The listing builds one solid part. Answer for the finished solid, in the listing's coordinates (mm). A direction names the side the tool comes from. Coordinates: 2 decimals unless noted, no trailing zeros. Loops run counter-clockwise (first coordinate to the right, second up) from the corner with the lowest first, then second, coordinate; pieces in that order, holes last. Notation, with made-up numbers: (-39.75, 73) - (-21.75, 73) arc R31 ccw to (-21.75, 109) - close; hole circle Ø10 at (-22.5, -10). An arc over 180 degrees is marked (long way). One line per question, with ' | ' between items.
from build123d import *

# Parameters (mm, degrees)
SKETCH_1_R      = 5
EXTRUDE_1_DEPTH = 10
CHAMFER_1_SIZE  = 1
SKETCH_2_R      = 4
EXTRUDE_2_DEPTH = 30
SKETCH_3_R      = 2
EXTRUDE_3_DEPTH = 10
FILLET_1_R      = 2


with BuildPart() as part:
    # Эскиз1 → Бобышка-Вытянуть1 (new body)
    with BuildSketch(Plane.XY):
        Circle(SKETCH_1_R)
    extrude(amount=EXTRUDE_1_DEPTH)

    # Фаска1
    chamfer_1_edges = [part.edges().sort_by_distance(p)[0] for p in [
        (-5, 0, 10),
    ]]
    chamfer(chamfer_1_edges, length=CHAMFER_1_SIZE)

    # Эскиз2 → Бобышка-Вытянуть2 (add)
    with BuildSketch(Plane.XY.offset(10)):
        Circle(SKETCH_2_R)
    extrude(amount=EXTRUDE_2_DEPTH)

    # Эскиз3 → Бобышка-Вытянуть3 (add)
    with BuildSketch(Plane.XY.offset(40)):
        Circle(SKETCH_3_R)
    extrude(amount=EXTRUDE_3_DEPTH)

    # Скругление1
    fillet_1_edges = [part.edges().sort_by_distance(p)[0] for p in [
        (-2, 0, 50),
    ]]
    fillet(fillet_1_edges, radius=FILLET_1_R)


solid = part.part
Item 1: Which of the six approach directions +Z, -Z, +X, -X, +Y, -Y give full straight-line access (tool end or side, diameter ignored) to faces 1 (the face through (0, -2, 44)), 2 (the face through (-1.08, -4.88, 4.44))?
Taken from the geometry:
face 1: +Z | face 2: +Z, -Z
Item 2: Find section A-A, the plane x = 0. Write down the section's boundary in (y, z), plus the area to 3 significant figures.
Taken from the geometry:
outline: (-5, 0) - (5, 0) - (5, 9) - (4, 10) - (4, 40) - (2, 40) - (2, 48) arc R2 ccw to (-2, 48) - (-2, 40) - (-4, 40) - (-4, 10) - (-5, 9) - close | area: 377 mm2
Item 3: Find the intervals of material crossed by line 1 (Z direction, x = 2, y = -3.25); line 2 (Y direction, x = 0, z = 16); line 3 (Y direction, x = 2.75, z = 4), in increasing order. Write a range as [from, to].
Taken from the geometry:
line 1: z = [0, 40] | line 2: y = [-4, 4] | line 3: y = [-4.18, 4.18]
Item 4: Each of these flat-tipped pins is pushed along its axis until it touches: pin 1 Ø3 at (x, z) = (-3.5, 31.5) entering from +Y; pin 2 Ø5 at (y, z) = (2, 11.5) entering from +X; pin 3 Ø1.5 at (y, z) = (-1, 13) entering from -X. Where does it stop, or does it pass through?
Taken from the geometry:
pin 1: stops at y = 3.46 | pin 2: stops at x = 4.72 | pin 3: stops at x = -3.99
Item 5: Find section B-B, the plane z = 11.5. Write down the section's boundary in (x, y), plus the area to 3 significant figures.
Taken from the geometry:
outline: circle Ø8 at (0, 0) | area: 50.3 mm2
Item 6: Find section C-C, the plane z = 5.5. Write down the section's boundary in (x, y), plus the area to 3 significant figures.
Taken from the geometry:
outline: circle Ø10 at (0, 0) | area: 78.5 mm2
